Autodesk Inventor part; units mm, degrees
ref_plane "YZ Plane" through (0, 0, 0) normal (1, 0, 0) x (0, 1, 0)
ref_plane "XZ Plane" through (0, 0, 0) normal (0, 1, 0) x (-1, 0, 0)
ref_plane "XY Plane" through (0, 0, 0) normal (0, 0, 1) x (1, 0, 0)
sketch "Sketch1" plane through (0, 0, 0) normal (0, 0, 1) x (1, 0, 0)
  line L0 (0, 0) -> (336.562362, 0)
  line L1 (336.562362, -12.7) -> (0, -12.7)
  line L2 (0, 0) -> (95.513688, 0)
  line L3 (95.513688, 0) -> (95.513688, -1.5875)
  line L4 (95.513688, -1.5875) -> (94.719938, -1.5875)
  line L5 (94.719938, -1.5875) -> (94.719938, 0)
  line L6 (95.513688, -1.5875) -> (96.307438, -1.5875)
  line L7 (96.307438, -1.5875) -> (96.307438, 0)
  line L8 (95.513688, -12.7) -> (95.513688, -11.1125)
  line L9 (95.513688, -11.1125) -> (94.719938, -11.1125)
  line L10 (94.719938, -11.1125) -> (94.719938, -12.7)
  line L11 (95.513688, -11.1125) -> (96.307438, -11.1125)
  line L12 (96.307438, -11.1125) -> (96.307438, -12.7)
  line L13 (336.562362, 0) -> (241.058362, 0)
  line L14 (241.058362, 0) -> (241.058362, -1.5875)
  line L15 (241.058362, -1.5875) -> (241.852112, -1.5875)
  line L16 (241.852112, -1.5875) -> (241.852112, 0)
  line L17 (241.058362, -1.5875) -> (240.264612, -1.5875)
  line L18 (240.264612, -1.5875) -> (240.264612, 0)
  line L19 (241.058362, -12.7) -> (241.058362, -11.1125)
  line L20 (241.058362, -11.1125) -> (241.852112, -11.1125)
  line L21 (241.852112, -11.1125) -> (241.852112, -12.7)
  line L22 (241.058362, -11.1125) -> (240.264612, -11.1125)
  line L23 (240.264612, -11.1125) -> (240.264612, -12.7)
  dimension "d1" = 91.9226
sketch "Sketch1 outline for Plate5" plane through (0, 0, 0) normal (0, 0, 1) x (1, 0, 0)
  line L0 (-91.9226, 0) -> (0, 0)
  line L1 (-91.9226, 12.7) -> (-91.9226, 0)
  line L2 (-84.4296, 12.7) -> (-91.9226, 12.7)
  line L3 (-42.418, 12.7) -> (-84.4296, 12.7)
  line L4 (0, 12.7) -> (-42.418, 12.7)
  line L5 (0, 0) -> (0, 12.7)
extrude "Plate5" add sketch "Sketch1 outline for Plate5" along normal blind 3.175
sketch "Sketch6" plane through (3.175, 0, -3.175) normal (1, 0, 0) x (0, 1, 0)
  line L0 (12.7, 0) -> (0, 0)
  line L1 (0, 0) -> (0, -138.3538)
  line L2 (0, -138.3538) -> (12.7, -138.3538)
  line L3 (12.7, -138.3538) -> (12.7, 0)
edge flange "Flange4" height 144.7038 angle 90 thickness 3.175 bend radius 3.175 thickness toward (1, 0, 0) relief tear relief width 3.175 relief depth 1.5875 edges at (0, 6.35, 0) wall of the first edge with corners at (3.175, 12.7, -3.175) (3.175, 0, -3.175) (3.175, 0, -141.5288) (3.175, 12.7, -141.5288)
bend "Bend4"
corner "Corner4"
sketch "Sketch7" plane through (0, 0, -144.7038) normal (0, 0, -1) x (-1, 0, 0)
  line L0 (0, 12.7) -> (0, 0)
  line L1 (0, 0) -> (91.9226, 0)
  line L2 (91.9226, 0) -> (91.9226, 12.7)
  line L3 (91.9226, 12.7) -> (0, 12.7)
edge flange "Flange5" height 98.2726 angle 90 thickness 3.175 bend radius 3.175 thickness toward (0, 0, -1) relief tear relief width 3.175 relief depth 1.5875 edges at (3.175, 6.35, -141.5288) wall of the first edge with corners at (0, 12.7, -144.7038) (0, 0, -144.7038) (-91.9226, 0, -144.7038) (-91.9226, 12.7, -144.7038)
bend "Bend5"
corner "Corner5"
sketch "Sketch9" plane through (0, 0, 3.175) normal (0, 0, 1) x (1, 0, 0)
  circle A0 centre (-42.4226, 501.2188) radius 3.3
  circle A1 centre (-84.4226, 501.2188) radius 3.3
extrude "Extrusion3" cut sketch "Sketch9" against normal blind 25374.6
sketch "Sketch10" plane through (-91.9226, 0, -144.7038) normal (0, 0, 1) x (1, 0, 0)
  line L0 (45, 276.1188) -> (45, -384.2812)
  circle A0 centre (7.5, 5.9188) radius 3.3
  circle A1 centre (49.5, 5.9188) radius 3.3
extrude "Extrusion4" cut sketch "Sketch10" along normal mid plane 25374.6
sketch "Sketch2" plane through (336.562362, -12.7, 0) normal (0, 0, 1) x (1, 0, 0)
  line L0 (-95.504, 12.7) -> (0, 12.7)
  line L1 (-95.504, 12.7) -> (-95.504, 11.1125)
  line L2 (-241.048674, 11.1125) -> (-241.048674, 12.7)
  line L3 (-336.562362, 12.7) -> (-241.048674, 12.7)
  line L4 (-241.048674, 12.7) -> (-241.842424, 12.7)
  line L5 (-241.842424, 12.7) -> (-241.842424, 11.1125)
  line L6 (-241.842424, 11.1125) -> (-241.048674, 11.1125)
  line L7 (-95.504, 12.7) -> (-94.71025, 12.7)
  line L8 (-95.504, 11.1125) -> (-94.71025, 11.1125)
  line L9 (-94.71025, 11.1125) -> (-94.71025, 12.7)
  dimension "d14" = 0.79375
  dimension "d15" = 0.79375
equation "\"d43\" = BendReliefWidth"
equation "\"d44\" = BendReliefDepth"
equation "\"d45\" = MinimumRemnant"
equation "\"d46\" = BendRadius"
equation "\"d49\" = BendRadius"
equation "\"d50\" = CornerReliefSize"
equation "\"d51\" = GapSize"
equation "\"d52\" = JacobiRadiusSize"
equation "\"d53\" = BendReliefWidth"
equation "\"d54\" = BendReliefDepth"
equation "\"d55\" = MinimumRemnant"
equation "\"d56\" = BendRadius"
equation "\"d59\" = BendRadius"
equation "\"d60\" = CornerReliefSize"
equation "\"d61\" = GapSize"
equation "\"d62\" = JacobiRadiusSize"
equation "\"BendRadius\" = Thickness"
equation "\"BendReliefWidth\" = Thickness"
equation "\"BendReliefDepth\" = 0.5 * Thickness"
equation "\"CornerReliefSize\" = 4 * Thickness"
equation "\"MinimumRemnant\" = 2 * Thickness"
equation "\"TransitionRadius\" = BendRadius"
equation "\"JacobiRadiusSize\" = BendRadius"
equation "\"GapSize\" = Thickness"
equation "\"d8\" = BendRadius"
equation "\"d42\" = BendRadius"
properties part number "tie-together tier 1" material "Aluminum 6061"
For this review, take the finished solid that the model builds, in its own axes (mm). A direction names the side the tool comes from. Give positions to 0.01 mm unless a question says otherwise; leave off trailing zeros. Loops run counter-clockwise (first coordinate to the right, second up) from the corner with the lowest first, then second, coordinate; pieces in that order, holes last. Notation, with made-up numbers: M 78,-4 L 137,-4 A16 cw 137,4 Z; hole C -31,-39 d5. An arc over 180 degrees is marked long. Answer as a JSON object with one key per item and string values. Group by question number.
Q1. Add section B-B on y = 11. Give the boundary of the cut face in (x, z) (3 decimals), and give its area (3 significant figures).
Q2. Add section D-D on z = -89.5. Give the boundary of the cut face in (x, y) (3 decimals).
Q3. Insertion check: P1, Ø4, axis at x = -42.42, y = 5.92, coming from the +Z side. The pin has a flat end and moves straight along its axis. Give the tip position at first contact, or say it passes through.
Q4. Mouldability with a two-part tool opening along Z and no side actions: class faces 1 (the cylindrical face through (2.22, 6.26, -143.8)), 2 (the flat face through (4, 12.7, -73)), 3 (the flat face through (-45, 9, -144.704)), 4 (the cylindrical face through (4.44, 6.26, -146.07)) as +Z half, -Z half, draft (parallel to the pull), parting line (faces both ways), or undercut.
Q5. Add section C-C on x = -41. Give the boundary of the cut face in (y, z) (3 decimals), and give its area (3 significant figures).
Q6. For probe 1 along Z at (x, y) = (-5, 4.75) (3 decimals); probe 2 along X at (y, z) = (12, -116.5) (3 decimals); probe 3 along Z at (x, y) = (1, 2.75), list the stretches that pass through material, from the lowest coordinate up. Write a range as [from, to].
Q7. Add section A-A on x = -26. Give the boundary of the cut face in (y, z) (3 decimals), and give its area (3 significant figures).
Q8. Tool access review of faces 5 (the flat face through (-47, 6, 0)), 6 (the flat face through (-47, 6, 3.175)): name each direction out of +Z, -Z, +X, -X, +Y, -Y from which nothing blocks a thin tool from reaching the whole face with its end or side.
Checked values:
{
 "1": {"outline": "M -91.923,-147.879 L 0,-147.879 A6.35 ccw 6.35,-141.529 L 6.35,-3.175 A6.35 ccw 0,3.175 L -91.923,3.175 L -91.923,0 L 0,0 A3.175 cw 3.175,-3.175 L 3.175,-141.529 A3.175 cw 0,-144.704 L -91.923,-144.704 Z", "area": "1,070 mm²"},
 "2": {"outline": "M 3.175,0 L 6.35,0 L 6.35,12.7 L 3.175,12.7 Z"},
 "3": {"P1": "through"},
 "4": {"face 1": "undercut", "face 2": "draft", "face 3": "undercut", "face 4": "-Z half"},
 "5": {"outline": "M 0,-147.879 L 2.941,-147.879 L 2.941,-144.704 L 0,-144.704 Z; M 0,0 L 2.941,0 L 2.941,3.175 L 0,3.175 Z; M 8.896,-147.879 L 12.7,-147.879 L 12.7,-144.704 L 8.896,-144.704 Z; M 8.896,0 L 12.7,0 L 12.7,3.175 L 8.896,3.175 Z", "area": "42.8 mm²"},
 "6": {"probe 1": "[-147.879, -144.704], [0, 3.175]", "probe 2": "[3.175, 6.35]", "probe 3": "[-147.8, -144.54], [-0.16, 3.1]"},
 "7": {"outline": "M 0,-147.879 L 12.7,-147.879 L 12.7,-144.704 L 0,-144.704 Z; M 0,0 L 12.7,0 L 12.7,3.175 L 0,3.175 Z", "area": "80.6 mm²"},
 "8": {"face 5": "-X, +Y, -Y", "face 6": "+Z, +X, -X, +Y, -Y"}
}
